Verification items for the finished model (mm, model axes). A direction names the side the tool comes from. Round coordinates to 2 decimals unless told otherwise and drop trailing zeros. Write each loop counter-clockwise with the first axis right and the second up, starting at its lowest first coordinate (ties: lowest second). Pieces come first, ordered by that corner, then holes. Notation, with made-up numbers: M -16,-12.75 L 22,-12.75 A18 cw 22,12.25 Z; hole C 31,-27 d10. An arc over 180 degrees is marked long. Write each question's results on one line, items separated by ' | '.
Autodesk Inventor part; units mm, degrees
ref_plane "YZ Plane" through (0, 0, 0) normal (1, 0, 0) x (0, 1, 0)
ref_plane "XZ Plane" through (0, 0, 0) normal (0, 1, 0) x (-1, 0, 0)
ref_plane "XY Plane" through (0, 0, 0) normal (0, 0, 1) x (1, 0, 0)
sketch "Sketch1" plane through (0, 0, 0) normal (0, 1, 0) x (-1, 0, 0)
  line L0 (0, 0) -> (-38.1, 0)
  line L1 (-38.1, 0) -> (-38.1, -114.3)
  line L2 (-38.1, -114.3) -> (0, -114.3)
  line L3 (0, -114.3) -> (0, 0)
  dimension "d0" = 38.1
  dimension "d1" = 114.3
extrude "Extrusion1" add sketch "Sketch1" along normal blind 3.175
sketch "Sketch3" plane through (0, 3.175, 0) normal (0, 1, 0) x (1, 0, 0)
  line L0 (31.75, 62.4332) -> (6.35, 62.4332)
  line L1 (6.35, 62.4332) -> (6.35, 37.0332)
  line L2 (6.35, 37.0332) -> (31.75, 37.0332)
  line L3 (31.75, 37.0332) -> (31.75, 62.4332)
  line L4 (38.1, 0) -> (38.1, 114.3)
  line L5 (38.1, 114.3) -> (0, 114.3)
  line L6 (28.575, 59.2582) -> (9.525, 59.2582)
  line L7 (9.525, 59.2582) -> (9.525, 40.2082)
  line L8 (9.525, 40.2082) -> (28.575, 40.2082)
  line L9 (28.575, 40.2082) -> (28.575, 59.2582)
  circle A0 centre (19.05, 49.7332) radius 2.54
  line L10 (0, 0) -> (38.1, 0)
  dimension "d8" = 25.4
  dimension "d9" = 25.4
  dimension "d10" = 6.35
  dimension "d12" = 3.175
  dimension "d15" = 5.08
  dimension "d16" = 12.7
  dimension "d17" = 12.7
  dimension "d23" = 37.0332
extrude "Extrusion3" add sketch "Sketch3" along normal blind 38.1 contours L3 L2 L1 L0
extrude "Extrusion5" cut sketch "Sketch3" against normal blind 3.175 contours A0
properties part number "mounting plate" material "ABS Plastic"
1) Depth check by flat-ended pin: P1, Ø1.5, axis at y = 4.5, z = -13, coming from the -X side; P2, Ø15, axis at x = 20.5, y = 17.5, coming from the -Z side; P3, Ø1.5, axis at x = 11.5, y = 33.5, coming from the +Z side; P4, Ø15, axis at y = 31.5, z = -50, coming from the +X side. Enter the tip coordinate at first touch or a pass-through.
Calculated:
P1: passes through | P2: stops at z = -62.43 | P3: stops at z = -37.03 | P4: stops at x = 31.75
2) Sectioned sample at D-D, the plane z = -82.5. Record the cut outline in (x, y) (3 decimals).
Calculated:
outline: M 0,0 L 38.1,0 L 38.1,3.175 L 0,3.175 Z
3) Sectioned sample at B-B, the plane x = 19.05. Record the cut outline in (y, z) (3 decimals), and give its area (3 significant figures).
Calculated:
outline: M 0,-114.3 L 3.175,-114.3 L 3.175,-62.433 L 41.275,-62.433 L 41.275,-59.258 L 3.175,-59.258 L 3.175,-52.273 L 0,-52.273 Z; M 0,-47.193 L 3.175,-47.193 L 3.175,-40.208 L 41.275,-40.208 L 41.275,-37.033 L 3.175,-37.033 L 3.175,0 L 0,0 Z | area: 589 mm²
4) Material ranges on line 1 (X direction, y = 7, z = -58) (3 decimals); line 2 (Z direction, x = 19.05, y = 2.4); line 3 (Z direction, x = 17, y = 14), recorded low to high. Write a range as [from, to].
Calculated:
line 1: x = [6.35, 9.525], [28.575, 31.75] | line 2: z = [-114.3, -52.27], [-47.19, 0] | line 3: z = [-62.43, -59.26], [-40.21, -37.03]
5) Access from +Z, -Z, +X, -X, +Y, -Y to the whole of each face (thin tool, end or side, straight path). Record for faces 1 (the flat face through (19, 22, -37.033)), 2 (the flat face through (19, 22, -59.258)), 3 (the flat face through (31.75, 22, -50)), 4 (the flat face through (6.35, 22, -50)), 5 (the flat face through (19, 22, -62.433)).
Calculated:
face 1: +Z, +X, -X, +Y | face 2: +Y | face 3: +Z, -Z, +X, +Y | face 4: +Z, -Z, -X, +Y | face 5: -Z, +X, -X, +Y
6) Sectioned sample at A-A, the plane y = 36.5. Record the cut outline in (x, z) (3 decimals), and give its area (3 significant figures).
Calculated:
outline: M 6.35,-62.433 L 31.75,-62.433 L 31.75,-37.033 L 6.35,-37.033 Z; hole M 9.525,-59.258 L 28.575,-59.258 L 28.575,-40.208 L 9.525,-40.208 Z | area: 282 mm²
7) Sectioned sample at C-C, the plane x = 8.5. Record the cut outline in (y, z) (3 decimals).
Calculated:
outline: M 0,-114.3 L 3.175,-114.3 L 3.175,-62.433 L 41.275,-62.433 L 41.275,-37.033 L 3.175,-37.033 L 3.175,0 L 0,0 Z
